from build123d import *

# Parameters (mm, degrees)
F0_W      = 50.518155098
F0_H      = 63.5085105896
F1_DEPTH  = 18
F2_DEPTH  = 496
F3_DEPTH  = 1996
F4_W      = 317.0488774776
F4_H      = 672.3350584507
F5_DEPTH  = 18
F6_DEPTH  = 66
F7_DEPTH  = 68
F8_DEPTH  = 6
F9_DEPTH  = 282
F10_DEPTH = 44
F11_DEPTH = 147
F12_W     = 357.6997369528
F12_H     = 883.1646442413
F13_DEPTH = 18
F14_DEPTH = 75
F15_DEPTH = 2


with BuildPart() as f1:
    # F0 (on Front) → F1 (new body)
    with BuildSketch(Plane.XZ):
        with Locations((25.259077549, 31.7542552948)):
            Rectangle(F0_W, F0_H)
    extrude(amount=F1_DEPTH)

    # F2 (add): a face of the model
    f2_faces = [f1.faces().sort_by_distance(p)[0] for p in [
        (0, -9, 31.7542552948),
    ]]
    extrude(f2_faces, amount=-F2_DEPTH)

    # F3 (add): a face of the model
    f3_faces = [f1.faces().sort_by_distance(p)[0] for p in [
        (248, -9, 0),
    ]]
    extrude(f3_faces, amount=-F3_DEPTH)

    # F4 (on face) → F5 (cut)
    with BuildSketch(Plane.XZ.offset(18)):
        with Locations((223.6920744181, 688.1462782621)):
            Rectangle(F4_W, F4_H)
    extrude(amount=-F5_DEPTH, mode=Mode.SUBTRACT)

    # F6 (add): a face of the model
    f6_faces = [f1.faces().sort_by_distance(p)[0] for p in [
        (65.1676356792, -9, 688.1462782621),
    ]]
    extrude(f6_faces, amount=F6_DEPTH)

    # F7 (cut): a face of the model
    f7_faces = [f1.faces().sort_by_distance(p)[0] for p in [
        (131.1676356792, -9, 688.1462782621),
    ]]
    extrude(f7_faces, amount=-F7_DEPTH, mode=Mode.SUBTRACT)

    # F8 (add): a face of the model
    f8_faces = [f1.faces().sort_by_distance(p)[0] for p in [
        (63.1676356792, -9, 688.1462782621),
    ]]
    extrude(f8_faces, amount=F8_DEPTH)

    # F9 (cut): a face of the model
    f9_faces = [f1.faces().sort_by_distance(p)[0] for p in [
        (225.6920744181, -9, 351.9787490368),
    ]]
    extrude(f9_faces, amount=-F9_DEPTH, mode=Mode.SUBTRACT)

    # F10 (cut): a face of the model
    f10_faces = [f1.faces().sort_by_distance(p)[0] for p in [
        (382.2165131569, -9, 547.1462782621),
    ]]
    extrude(f10_faces, amount=-F10_DEPTH, mode=Mode.SUBTRACT)

    # F11 (add): a face of the model
    f11_faces = [f1.faces().sort_by_distance(p)[0] for p in [
        (247.6920744181, -9, 1024.3138074875),
    ]]
    extrude(f11_faces, amount=F11_DEPTH)

    # F12 (on face) → F13 (cut)
    with BuildSketch(Plane.XZ.offset(18)):
        with Locations((249.6171072125, 1463.1779193878)):
            Rectangle(F12_W, F12_H)
    extrude(amount=-F13_DEPTH, mode=Mode.SUBTRACT)

    # F14 (cut): a face of the model
    f14_faces = [f1.faces().sort_by_distance(p)[0] for p in [
        (249.6171072125, -9, 1021.5955972672),
    ]]
    extrude(f14_faces, amount=-F14_DEPTH, mode=Mode.SUBTRACT)

    # F15 (add): a face of the model
    f15_faces = [f1.faces().sort_by_distance(p)[0] for p in [
        (428.4669756889, -9, 1425.6779193878),
    ]]
    extrude(f15_faces, amount=F15_DEPTH)


solid = f1.part
Verification items for the finished model (mm, model axes). Round coordinates to 2 decimals unless told otherwise and drop trailing zeros. Order: outer loops, then holes, each group sorted by start corner. A loop starts at its lowest first (then second) coordinate and runs counter-clockwise, first axis right, second up.
1. Section check D-D on z = 1522. Record the cut outline in (x, y).
Final values:
outline: (0, -18) - (70.77, -18) - (70.77, 0) - (0, 0) - close; (426.47, -18) - (496, -18) - (496, 0) - (426.47, 0) - close
2. Section check C-C on x = 370.5. Record the cut outline in (y, z).
Final values:
outline: (-18, 0) - (0, 0) - (0, 69.98) - (-18, 69.98) - close; (-18, 877.31) - (0, 877.31) - (0, 946.6) - (-18, 946.6) - close; (-18, 1904.76) - (0, 1904.76) - (0, 1996) - (-18, 1996) - close
3. Section check A-A on z = 313. Record the cut outline in (x, y).
Final values:
outline: (0, -18) - (69.17, -18) - (69.17, 0) - (0, 0) - close; (426.22, -18) - (496, -18) - (496, 0) - (426.22, 0) - close
4. Thickness scan on L1, parallel to Z at x = 220.5, y = -4; L2, parallel to X at y = -16, z = 843; L3, parallel to X at y = -14, z = 1260.5. Record the ranges inside material, lowest first.
Final values:
L1: z = 0 to 69.98, 877.31 to 946.6, 1904.76 to 1996
L2: x = 0 to 69.17, 426.22 to 496
L3: x = 0 to 70.77, 426.47 to 496
5. Section check B-B on y = -11.5. Record the cut outline in (x, z).
Final values:
outline: (0, 0) - (496, 0) - (496, 1996) - (0, 1996) - close; hole (69.17, 69.98) - (426.22, 69.98) - (426.22, 877.31) - (69.17, 877.31) - close; hole (70.77, 946.6) - (426.47, 946.6) - (426.47, 1904.76) - (70.77, 1904.76) - close
